Read the model definition and answer for the solid it produces. Units are mm, in the model's axes. Face numbers are marked on the shaded views. A direction names the side the tool comes from. Give positions to 0.01 mm unless a question says otherwise; leave off trailing zeros. Loops run counter-clockwise (first coordinate to the right, second up) from the corner with the lowest first, then second, coordinate; pieces in that order, holes last. Notation, with made-up numbers: (-2, 25) - (44, 25) arc R23 ccw to (44, 45) - close; hole circle Ø6 at (-6, 63.5). An arc over 180 degrees is marked (long way). Put each result on its own line as item: value. Start each with the question number.
1. Given pin 1 Ø1.5 at (y, z) = (-6, 121) entering from +X; pin 2 Ø6 at (y, z) = (-6.5, 40.5) entering from -X; pin 3 Ø2 at (y, z) = (8.5, 53.5) entering from -X, each flat-ended and moving along its own axis, determine where each tip first touches the part or whether it passes through.
2. A cutting plane is placed at C-C, the plane z = 8.5. Determine the outline of the cut face in (x, y).
3. A cutting plane is placed at A-A, the plane y = 0. Determine the outline of the cut face in (x, z).
4. A cutting plane is placed at D-D, the plane x = -8.25. Determine the outline of the cut face in (y, z).
5. Consider L1, parallel to Z at x = -10.5, y = 0.75; L2, parallel to X at y = 11, z = 18; L3, parallel to X at y = -0.5, z = 35. Determine where each line is inside the solid, lowest interval first. Write a range as from..to.
6. For the marked faces 1, 2 and 3, determine the directions among +Z, -Z, +X, -X, +Y, -Y from which every point of the face is accessible in a straight line to the end or side of a thin tool.
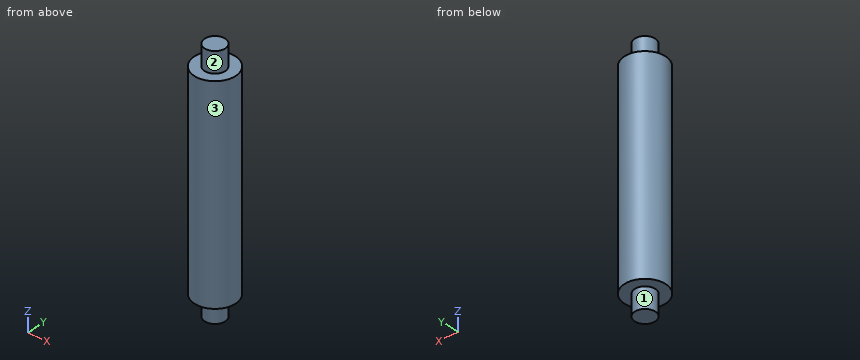
```python
from build123d import *

# Parameters (mm, degrees)
SKETCH1_W   = 12.7
SKETCH1_H   = 6.35
SKETCH1_W_2 = 127.762
SKETCH1_H_2 = 12.7


with BuildPart() as part:
    # Sketch1 → Revolve1 (revolve)
    with BuildSketch(Plane(origin=(0, 0, 0), x_dir=(0, 0, -1), z_dir=(1, 0, 0))):
        with Locations((-134.112, 3.175)):
            Rectangle(SKETCH1_W, SKETCH1_H)
        with Locations((-63.881, 6.35)):
            Rectangle(SKETCH1_W_2, SKETCH1_H_2)
        with Locations((6.35, 3.175)):
            Rectangle(SKETCH1_W, SKETCH1_H)
    revolve(axis=Axis((0, 0, 0), (0, 0, 1)))


solid = part.part
```
Return value:
1. pin 1: stops at x = 11.56
1. pin 2: stops at x = -12.21
1. pin 3: stops at x = -10.25
2. outline: circle Ø25.4 at (0, 0)
3. outline: (-12.7, 0) - (-6.35, 0) - (-6.35, -12.7) - (6.35, -12.7) - (6.35, 0) - (12.7, 0) - (12.7, 127.76) - (6.35, 127.76) - (6.35, 140.46) - (-6.35, 140.46) - (-6.35, 127.76) - (-12.7, 127.76) - close
4. outline: (-9.66, 0) - (9.66, 0) - (9.66, 127.76) - (-9.66, 127.76) - close
5. L1: z = 0..127.76
5. L2: x = -6.35..6.35
5. L3: x = -12.69..12.69
6. face 1: -Z
6. face 2: +Z
6. face 3: +Z, -Z
